Source: CAD feature listing. Evaluate the final solid. Frame: model axes, mm. A direction names the side the tool comes from. Give positions to 0.01 mm unless a question says otherwise; leave off trailing zeros. Loops run counter-clockwise (first coordinate to the right, second up) from the corner with the lowest first, then second, coordinate; pieces in that order, holes last. Notation, with made-up numbers: M 88,57.5 L 96,57.5 A25 cw 96,91.5 Z; hole C 10.5,29 d11. An arc over 180 degrees is marked long. Answer in a Markdown table with one row per item.
```python
from build123d import *

# Parameters (mm, degrees)
F1_DEPTH  = 67
F3_DEPTH  = 70.001
F4_W      = 36
F4_H      = 12.5
F5_DEPTH  = 25
F6_W      = 3
F6_H      = 43
F7_DEPTH  = 2
F8_W      = 1.6
F8_H      = 33
F9_DEPTH  = 6.001
F10_W     = 42
F10_H     = 4
F11_DEPTH = 13
F13_SIZE  = 5
F14_SIZE  = 3.99999
F15_SIZE  = 15
F16_SIZE  = 7
F12_R     = 3
F17_DEPTH = 71.001
F18_W     = 30
F18_H     = 45
F19_DEPTH = 3
F20_SIZE  = 2.99999
F21_SIZE  = 2
F22_SIZE2 = 1.5
F22_SIZE  = 2.5
F24_START = -43
F23_W     = 62
F23_H     = 16.8932331726
F24_DEPTH = 57


# Not quite as in the source:
# - a fillet or chamfer is up to 0.001 mm smaller than in the source, because OpenCascade refuses the exact size


with BuildPart() as f1:
    # F0 (on Front) → F1 (new body)
    with BuildSketch(Plane.XZ):
        Polygon((35, 0), (-35, 0), (-35, -19), (-27, -19), (-27, -16), (-31, -12), (-31, -4), (31, -4), (31, -12), (27, -16), (27, -19), (35, -19), align=None)
    extrude(amount=F1_DEPTH)

    # F2 (on face) → F3 (cut, through all)
    with BuildSketch(Plane.YZ.offset(35)):
        with BuildLine():
            Line((-13.190586324, -6.5416721678), (-19, -19))
            Line((-19, -19), (4.1351475573, -19))
            Line((4.1351475573, -19), (4.1351475573, -2.5))
            Line((4.1351475573, -2.5), (-6.8464318148, -2.5))
            ThreePointArc((-6.8464318148, -2.5), (-10.6075290732, -3.5962598793), (-13.190586324, -6.5416721678))
        make_face()
    extrude(amount=-F3_DEPTH, mode=Mode.SUBTRACT)

    # F4 (on face) → F5 (cut)
    with BuildSketch(Plane.XY):
        with Locations((0, -12.75)):
            Rectangle(F4_W, F4_H)
    extrude(amount=-F5_DEPTH, mode=Mode.SUBTRACT)

    # F6 (on face) → F7 (join)
    with BuildSketch(Plane(origin=(0, 0, -4), x_dir=(1, 0, 0), z_dir=(0, 0, -1))):
        with Locations((-19.5, 45.5)):
            Rectangle(F6_W, F6_H)
        with Locations((19.5, 45.5)):
            Rectangle(F6_W, F6_H)
    extrude(amount=F7_DEPTH)

    # F8 (on face) → F9 (cut, through all)
    with BuildSketch(Plane(origin=(0, 0, -6), x_dir=(1, 0, 0), z_dir=(0, 0, -1))):
        with Locations((-19.5, 44.5)):
            Rectangle(F8_W, F8_H)
        with Locations((19.5, 44.5)):
            Rectangle(F8_W, F8_H)
    extrude(amount=-F9_DEPTH, mode=Mode.SUBTRACT)

    # F10 (on face) → F11 (join)
    with BuildSketch(Plane.XY):
        with Locations((0, -69)):
            Rectangle(F10_W, F10_H)
    extrude(amount=-F11_DEPTH)

    # F13
    f13_edges = [f1.edges().sort_by_distance(p)[0] for p in [
        (-35, -43, -19),
        (35, -43, -19),
    ]]
    chamfer(f13_edges, length=F13_SIZE)

    # F14 (size 4 in the source; OpenCascade refuses exactly that, so slightly less here)
    f14_edges = [f1.edges().sort_by_distance(p)[0] for p in [
        (-21, -67, -2),
        (21, -67, -2),
    ]]
    chamfer(f14_edges, length=F14_SIZE)

    # F15
    f15_edges = [f1.edges().sort_by_distance(p)[0] for p in [
        (35, 0, -1.25),
        (-35, 0, -1.25),
    ]]
    chamfer(f15_edges, length=F15_SIZE)

    # F16
    f16_edges = [f1.edges().sort_by_distance(p)[0] for p in [
        (-21, -69, -13),
        (21, -69, -13),
    ]]
    chamfer(f16_edges, length=F16_SIZE)

    # F12 (on face) → F17 (cut, through all)
    with BuildSketch(Plane.XZ.offset(71)):
        with Locations((0, -8)):
            Circle(F12_R)
    extrude(amount=-F17_DEPTH, mode=Mode.SUBTRACT)

    # F18 (on face) → F19 (cut)
    with BuildSketch(Plane(origin=(0, 0, -4), x_dir=(1, 0, 0), z_dir=(0, 0, -1))):
        with Locations((0, 44.5)):
            Rectangle(F18_W, F18_H)
    extrude(amount=-F19_DEPTH, mode=Mode.SUBTRACT)

    # F20 (size 3 in the source; OpenCascade refuses exactly that, so slightly less here)
    f20_edges = [f1.edges().sort_by_distance(p)[0] for p in [
        (0, -67, -1),
        (-15, -44.5, -1),
        (0, -22, -1),
        (15, -44.5, -1),
    ]]
    chamfer(f20_edges, length=F20_SIZE)

    # F21
    f21_edges = [f1.edges().sort_by_distance(p)[0] for p in [
        (20.3, -44.5, 0),
        (18.7, -44.5, 0),
        (19.5, -28, 0),
        (19.5, -61, 0),
        (-18.7, -44.5, 0),
        (-19.5, -28, 0),
        (-19.5, -61, 0),
        (-20.3, -44.5, 0),
    ]]
    chamfer(f21_edges, length=F21_SIZE)

    # F22
    f22_edges = [f1.edges().sort_by_distance(p)[0] for p in [
        (0, 0, -2.5),
    ]]
    f22_side = f1.faces().sort_by_distance((0, -3.465238, -2.5))[0]
    chamfer(f22_edges, length=F22_SIZE, length2=F22_SIZE2, reference=f22_side)

    # F23 (on face) → F24 (cut)
    with BuildSketch(Plane.XZ.offset(67).offset(F24_START)):
        with Locations((0, -17.7232683636)):
            Rectangle(F23_W, F23_H)
    extrude(amount=-F24_DEPTH, mode=Mode.SUBTRACT)


solid = f1.part
```
Q1. Ray query, probe 1 along Z at (x, y) = (0, -68.8); probe 2 along X at (y, z) = (-47.5, -12); probe 3 along X at (y, z) = (-60, -1.75). Return the intervals inside material, ascending. Write a range as from..to.
Values follow:
| item | result |
|---|---|
| probe 1 | -13..-11, -5..0 |
| probe 2 | -35..-31, 31..35 |
| probe 3 | -35..-20.55, -18.45..-12.75, 12.75..18.45, 20.55..35 |
Q2. Mould query, pull axis Z, two halves, no side actions, for faces 1 (the cylindrical face through (-23.801, -8.963, -2.828)), 2 (the flat face through (-20, -24, -5)), 3 (the flat face through (31, -39, -8)). Classes: +Z half, -Z half, draft (parallel to the pull), parting line (faces both ways), or undercut.
Values follow:
| item | result |
|---|---|
| face 1 | -Z half |
| face 2 | draft |
| face 3 | undercut |
Q3. Reachability of faces 4 (the flat face through (-20, -62, -1)), 5 (the flat face through (-31.2, -67, -7.3)), 6 (the flat face through (-18, -13, -2)), 7 (the flat face through (-29, -24, -16)), 8 (the flat face through (27, -45, -17)) from +Z, -Z, +X, -X, +Y, -Y: full face, straight path, thin tool, end or side. Return the list, or none.
Values follow:
| item | result |
|---|---|
| face 4 | +Z |
| face 5 | +Z, -Z, -X, -Y |
| face 6 | +Z, -Z |
| face 7 | -Z, +Y |
| face 8 | -Z, +Y, -Y |
Q4. Contact query for flat-ended pins moving along their axis: pin 1 Ø1.5 at (x, y) = (20.5, -39) entering from +Z; pin 2 Ø4.5 at (x, z) = (-30, -15) entering from +Y; pin 3 Ø8 at (x, y) = (-9, -51.5) entering from -Z; pin 4 Ø6 at (x, y) = (-19.5, -38) entering from +Z. Output: stop coordinate, or through.
Values follow:
| item | result |
|---|---|
| pin 1 | z = -1.05 |
| pin 2 | y = -16.19 |
| pin 3 | z = -2 |
| pin 4 | z = 0 |
Q5. Section query A-A (x = 0). Give the number of separate pieces and of enclosed holes in the cut face, plus the area to 3 significant figures.
Values follow:
| item | result |
|---|---|
| separate pieces | 3 |
| enclosed holes | 0 |
| area | 108 mm^2 |
Q6. Section query C-C (z = -8). Output: boundary loops of the cut face in (x, y), plus the area to 3 significant figures.
Values follow:
| item | result |
|---|---|
| outline | M -35,-67 L -31,-67 L -31,-13.87 L -33.87,-13.87 L -35,-15 Z; M -19,-71 L -3,-71 L -3,-67 L -19,-67 Z; M 3,-71 L 19,-71 L 19,-67 L 3,-67 Z; M 31,-67 L 35,-67 L 35,-15 L 33.87,-13.87 L 31,-13.87 Z |
| area | 552 mm^2 |
